Part model, mm, in its own coordinate system. Face numbers are marked on the shaded views. A direction names the side the tool comes from. Coordinates: 2 decimals unless noted, no trailing zeros. Order: outer loops, then holes, each group sorted by start corner. A loop starts at its lowest first (then second) coordinate and runs counter-clockwise, first axis right, second up.
1) Wall check: L1, parallel to Z at x = -129, y = 177.5; L2, parallel to X at y = 0, z = -17; L3, parallel to Y at x = 5, z = -17.5. Give the ranges that are in metal, low to high.
2) Pin check, flat tips, straight feed: pin 1 Ø1 at (x, z) = (-49.5, 6.5) entering from +Y; pin 2 Ø1 at (y, z) = (-108.5, 2.5) entering from -X; pin 3 Ø2 at (y, z) = (-70, -15) entering from +X. Stop position of each tip, or through.
3) Cut at C-C (y = -61). List the corners of the cut face in (x, z).
4) Cut at D-D (z = -6). List the corners of the cut face in (x, y), and give its area (3 significant figures).
5) Cut at A-A (z = 22). List the corners of the cut face in (x, y).
6) Mould opens along Y. For the marked faces 1, 2 and 3 say: +Y half, -Y half, draft (parallel to the pull), parting line (faces both ways), or undercut.
7) Cut at B-B (x = 53.5). List the corners of the cut face in (y, z), and give its area (3 significant figures).
8) Tool access for the marked faces 4, 5 and 6: list every direction of +Z, -Z, +X, -X, +Y, -Y with a clear straight run to the whole face (end or side of a thin tool).
```python
from build123d import *

# Parameters (mm, degrees)
SKETCH2_R           = 90
BOSS_EXTRUDE1_DEPTH = 60.865268403


with BuildPart() as part:
    # Sketch1 → Revolve1 (revolve)
    with BuildSketch(Plane(origin=(0, 0, 0), x_dir=(1, 0, 0), z_dir=(0, 1, 0))):
        Polygon((-90, -29.79575879), (-90, -14.79575879), (-70, -14.79575879), (-70, 48.140410311), (-99.097023169, 48.140410311), (-99.097023169, 31.069509613), (-158.113565582, 31.069509613), (-158.113565582, -29.79575879), align=None)
    revolve(axis=Axis((0, 0, 0), (0, 0, 1)))

    # Sketch2 → Boss-Extrude1 (add)
    with BuildSketch(Plane(origin=(0, 0, -31.069509613), x_dir=(-1, 0, 0), z_dir=(0, 0, -1))):
        with BuildLine():
            Line((0, -158.113565582), (341.027566012, -158.113565582))
            Line((341.027566012, -158.113565582), (341.027566012, -116.806868092))
            Line((341.027566012, -116.806868092), (233.535117418, -116.806868092))
            Line((233.535117418, -116.806868092), (194.760807878, -46.320749515))
            ThreePointArc((194.760807878, -46.320749515), (176.203837582, 23.778561234), (192.69826547, 94.391650408))
            Line((192.69826547, 94.391650408), (255.959925105, 217.8266932))
            Line((255.959925105, 217.8266932), (206.159608852, 243.349839506))
            Line((206.159608852, 243.349839506), (179.847269567, 192.009663729))
            Line((179.847269567, 192.009663729), (-27.270239804, 155.744128756))
            ThreePointArc((-27.270239804, 155.744128756), (-157.520092587, -13.686491605), (0, -158.113565582))
        make_face()
        Circle(SKETCH2_R, mode=Mode.SUBTRACT)
    extrude(amount=-BOSS_EXTRUDE1_DEPTH)


solid = part.part
```
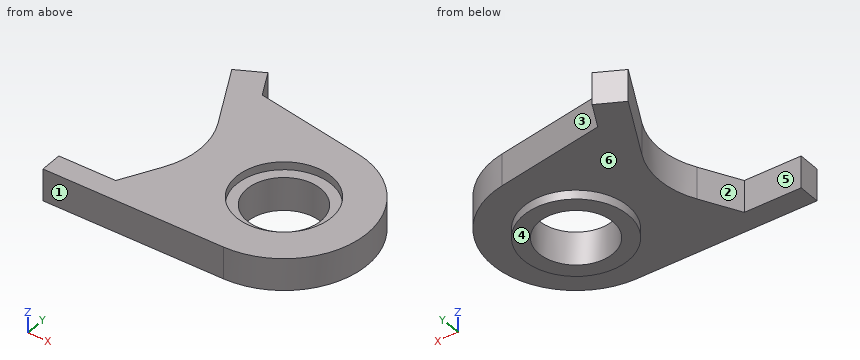
Geometry check:
1. L1: z = -31.07 to 29.8
1. L2: x = -178.45 to -70, 70 to 158.11
1. L3: y = -158.03 to -69.82, 69.82 to 159.64
2. pin 1: stops at y = 169.27
2. pin 2: stops at x = -229.24
2. pin 3: stops at x = 142.26
3. outline: (-202.84, -31.07) - (-78.1, -31.07) - (-78.1, -48.14) - (-34.34, -48.14) - (-34.34, 14.8) - (-66.17, 14.8) - (-66.17, 29.8) - (-202.84, 29.8) - close; (34.34, -48.14) - (78.1, -48.14) - (78.1, -31.07) - (145.87, -31.07) - (145.87, 29.8) - (66.17, 29.8) - (66.17, 14.8) - (34.34, 14.8) - close
4. outline: (-341.03, -158.11) - (0, -158.11) arc R158.11 ccw to (27.27, 155.74) - (-179.85, 192.01) - (-206.16, 243.35) - (-255.96, 217.83) - (-192.7, 94.39) arc R150 cw to (-194.76, -46.32) - (-233.54, -116.81) - (-341.03, -116.81) - close; hole circle Ø140 at (0, 0)
4. area: 99,500 mm2
5. outline: (-341.03, -158.11) - (0, -158.11) arc R158.11 ccw to (27.27, 155.74) - (-179.85, 192.01) - (-206.16, 243.35) - (-255.96, 217.83) - (-192.7, 94.39) arc R150 cw to (-194.76, -46.32) - (-233.54, -116.81) - (-341.03, -116.81) - close; hole circle Ø180 at (0, 0)
6. face 1: -Y half
6. face 2: undercut
6. face 3: +Y half
7. outline: (-148.79, -31.07) - (-83.41, -31.07) - (-83.41, -48.14) - (-45.14, -48.14) - (-45.14, 14.8) - (-72.37, 14.8) - (-72.37, 29.8) - (-148.79, 29.8) - close; (45.14, -48.14) - (83.41, -48.14) - (83.41, -31.07) - (148.79, -31.07) - (148.79, 29.8) - (72.37, 29.8) - (72.37, 14.8) - (45.14, 14.8) - close
7. area: 13,100 mm2
8. face 4: -Z, +X, -X, +Y, -Y
8. face 5: +Z, -Z, -X
8. face 6: -Z
